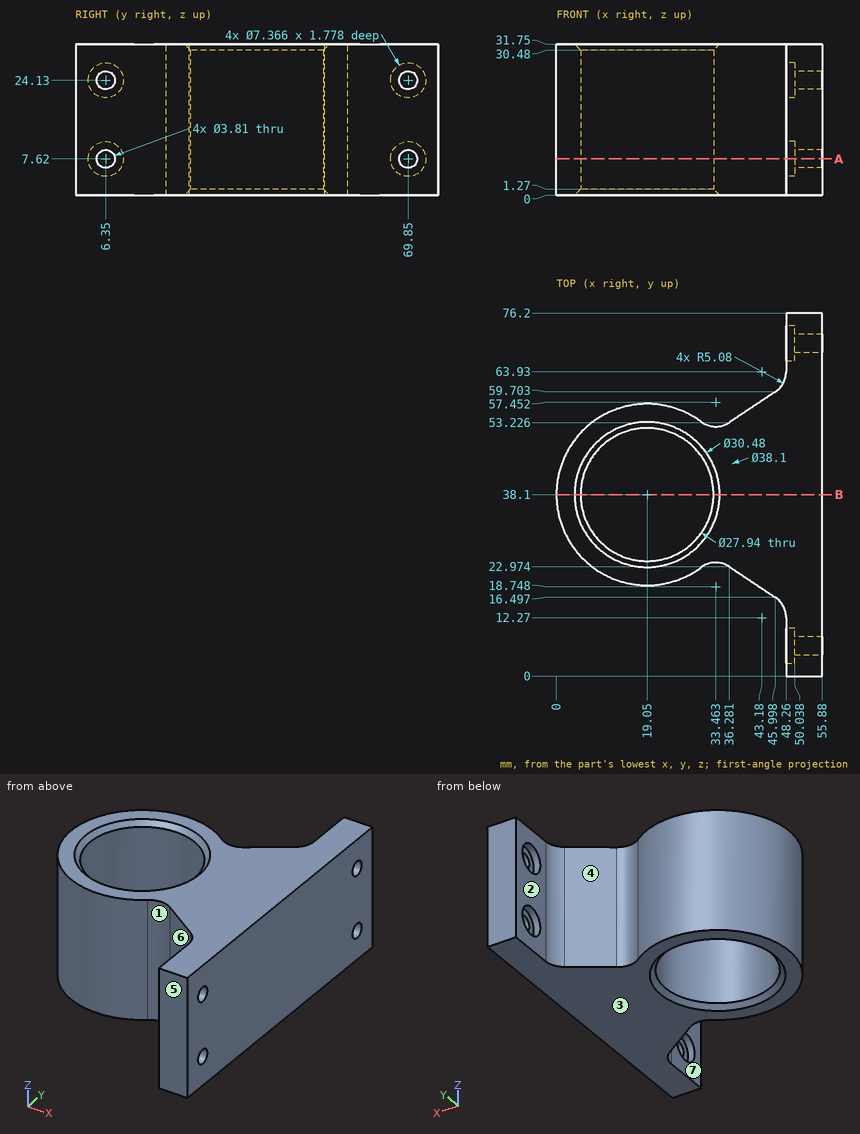
Source: three-view drawing plus pictorial views. Frame: mm from the lowest corner of the part. A direction names the side the tool comes from. Coordinates: 2 decimals unless noted, no trailing zeros. Loops run counter-clockwise (first coordinate to the right, second up) from the corner with the lowest first, then second, coordinate; pieces in that order, holes last. Notation, with made-up numbers: M 70,-32.5 L 90,-32.5 A26 ccw 90,-14.5 Z; hole C -0.75,43.5 d6. An arc over 180 degrees is marked long. Use CSV: the item, a comma, the result in double quotes.
(1) Line query: line 1 (Y direction, x = 19, z = 19); line 2 (Y direction, x = 48.5, z = 23) (1 decimal); line 3 (X direction, y = 71.5, z = 3.5). Output: solid intervals per line, ascending. Write a range as [from, to].
Answers follow:
line 1,"[19.05, 24.13], [52.07, 57.15]"
line 2,"[0, 2.8], [9.9, 66.3], [73.4, 76.2]"
line 3,"[48.26, 55.88]"
(2) Cut plane A-A on z = 7.62. Give the number of separate pieces and of enclosed holes in the cut face, and give its area (3 significant figures).
Answers follow:
separate pieces,"3"
enclosed holes,"1"
area,"1,500 mm²"
(3) Reachability of the marked faces 4, 5, 6 and 7 from +Z, -Z, +X, -X, +Y, -Y: full face, straight path, thin tool, end or side. Return the list, or none.
Answers follow:
face 4,"+Z, -Z, +Y"
face 5,"+Z, -Z, +X, -X, -Y"
face 6,"+Z, -Z, -Y"
face 7,"+Z, -Z, -X, -Y"
(4) Contact query for flat-ended pins moving along their axis: pin 1 (6 mm diameter, centred on x = 41, z = 5, fed in from +Y); pin 2 (2 mm diameter, centred on y = 70.5, z = 24, fed in from -X); pin 3 (3.5 mm diameter, centred on y = 7.5, z = 23, fed in from -X); pin 4 (10 mm diameter, centred on y = 68.5, z = 13, fed in from -X). Output: stop coordinate, or through.
Answers follow:
pin 1,"y = 58.37"
pin 2,"through"
pin 3,"x = 50.04"
pin 4,"x = 48.24"
(5) Draft query along X for the marked faces 1, 2 and 3. Return one class per face: pulls with the +X half, pulls with the -X half, needs draft (parallel to the pull), parting line crosses it, or undercut.
Answers follow:
face 1,"undercut"
face 2,"pulls with the -X half"
face 3,"needs draft"
(6) Cut plane B-B on y = 38.1. Return loops of the section in (x, z), and give its area (3 significant figures).
Answers follow:
outline,"M 0,0 L 3.81,0 L 5.08,1.27 L 5.08,30.48 L 3.81,31.75 L 0,31.75 Z; M 33.02,1.27 L 34.29,0 L 55.88,0 L 55.88,31.75 L 34.29,31.75 L 33.02,30.48 Z"
area,"884 mm²"
